from build123d import *

# Parameters (mm, degrees)
F0_R     = 15.875
F1_DEPTH = 28.575
F2_R     = 6.35
F3_DEPTH = 44.45
F4_R     = 4.445
F5_DEPTH = 76.2


with BuildPart() as f1:
    # F0 (on Top) → F1 (new body)
    with BuildSketch(Plane.XY):
        Circle(F0_R)
    extrude(amount=F1_DEPTH)

    # F2 (on face) → F3 (join)
    with BuildSketch(Plane(origin=(0, 0, 0), x_dir=(1, 0, 0), z_dir=(0, 0, -1))):
        Circle(F2_R)
    extrude(amount=F3_DEPTH)

    # F4 (on Right) → F5 (join, symmetric)
    with BuildSketch(Plane.YZ):
        with Locations((0, 12.7)):
            Circle(F4_R)
    extrude(amount=F5_DEPTH, both=True)

    # F6 (on Front) → F7 (revolve)
    with BuildSketch(Plane.XZ):
        with BuildLine():
            Line((-86.433909, 12.7), (-66.113909, 12.7))
            ThreePointArc((-66.113909, 12.7), (-76.273909, 22.86), (-86.433909, 12.7))
        make_face()
        with BuildLine():
            ThreePointArc((86.433909, 12.7), (76.273909, 22.86), (66.113909, 12.7))
            Line((66.113909, 12.7), (86.433909, 12.7))
        make_face()
    revolve(axis=Axis((-66.812286, 0, 12.7), (1, 0, 0)))


solid = f1.part
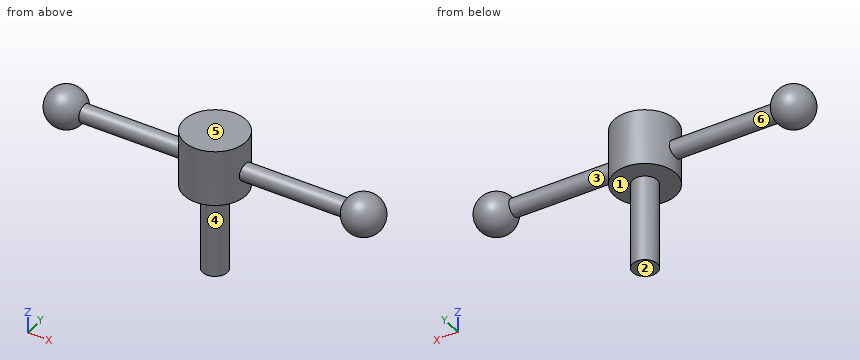
The model under review builds one solid part; all positions refer to its coordinate system, in mm. Face numbers are marked on the shaded views. A direction names the side the tool comes from. Round coordinates to 2 decimals unless told otherwise and drop trailing zeros. Order: outer loops, then holes, each group sorted by start corner. A loop starts at its lowest first (then second) coordinate and runs counter-clockwise, first axis right, second up. Notation, with made-up numbers: (-36, 28) - (20, 28) arc R29 ccw to (20, 54) - close; hole circle Ø6 at (60.5, 74). An arc over 180 degrees is marked (long way). Use one line per item in the form item = value.
Q1. Tool access review of the marked faces 1, 2 and 3: name each direction out of +Z, -Z, +X, -X, +Y, -Y from which nothing blocks a thin tool from reaching the whole face with its end or side.
Response values:
face_1 = -Z
face_2 = -Z, +X, -X, +Y, -Y
face_3 = none
Q2. To check wall thickness, follow line 1 (X direction, y = 5.5, z = 9.5); line 2 (X direction, y = 7, z = 6.5); line 3 (Z direction, x = -7, y = 14) (3 decimals). State the ranges of each line that lie inside material, in increasing order.
Response values:
line_1 = -84.19 to -68.35, -14.89 to 14.89, 68.35 to 84.19
line_2 = -80.25 to -72.3, -14.25 to 14.25, 72.3 to 80.25
line_3 = 0 to 28.575
Q3. Add section B-B on y = 0. Give the boundary of the cut face in (x, z) (3 decimals), then the cut area to 3 significant figures.
Response values:
outline = (-67.138, 8.255) - (-15.875, 8.255) - (-15.875, 0) - (-6.35, 0) - (-6.35, -44.45) - (6.35, -44.45) - (6.35, 0) - (15.875, 0) - (15.875, 8.255) - (67.138, 8.255) arc R10.16 ccw (long way) to (67.138, 17.145) - (15.875, 17.145) - (15.875, 28.575) - (-15.875, 28.575) - (-15.875, 17.145) - (-67.138, 17.145) arc R10.16 ccw (long way) to start
area = 3,020 mm^2
Q4. Add section C-C on x = 0. Give the boundary of the cut face in (y, z) (3 decimals).
Response values:
outline = (-15.875, 0) - (-6.35, 0) - (-6.35, -44.45) - (6.35, -44.45) - (6.35, 0) - (15.875, 0) - (15.875, 28.575) - (-15.875, 28.575) - close
Q5. Mouldability with a two-part tool opening along X and no side actions: class the marked faces 4, 5 and 6 as pulls with the +X half, pulls with the -X half, needs draft (parallel to the pull), parting line crosses it, or undercut.
Response values:
face_4 = parting line crosses it
face_5 = needs draft
face_6 = undercut
Q6. Add section D-D on z = 21. Give the boundary of the cut face in (x, y) (3 decimals).
Response values:
outline = circle Ø11.719 at (-76.274, 0); circle Ø31.75 at (0, 0); circle Ø11.719 at (76.274, 0)
Q7. Add section A-A on z = 12.7. Give the boundary of the cut face in (x, y) (3 decimals).
Response values:
outline = (-67.138, -4.445) - (-15.24, -4.445) arc R15.875 ccw to (15.24, -4.445) - (67.138, -4.445) arc R10.16 ccw (long way) to (67.138, 4.445) - (15.24, 4.445) arc R15.875 ccw to (-15.24, 4.445) - (-67.138, 4.445) arc R10.16 ccw (long way) to start
Q8. Clearance check with flat-ended pins moving along their axes: P1, Ø12, axis at y = 12.5, z = 8, coming from the +X side; P2, Ø2, axis at y = 3, z = -19.5, coming from the +X side. State where each tip first meets the part, or that it passes through.
Response values:
P1 = 83.28
P2 = 6.03
